Check sheet for the modelled part. Datum: model origin and axes. Units: mm. Give positions to 0.01 mm unless a question says otherwise; leave off trailing zeros. Order: outer loops, then holes, each group sorted by start corner. A loop starts at its lowest first (then second) coordinate and runs counter-clockwise, first axis right, second up. Notation, with made-up numbers: (28, -21) -> (55, -21) arc R27 ccw to (55, 6) -> close; hole circle Ø6 at (41, -30). An arc over 180 degrees is marked (long way). Answer in a Markdown table with one row per item. Add a question column.
(1) Cross-section at A-A (x = 10.5). Record the cut outline in (y, z).
(2) Cross-section at B-B (y = 21). Record the cut outline in (x, z), then the cut area to 3 significant figures.
(3) Cross-section at D-D (z = 0). Record the cut outline in (x, y).
(4) Release check for a two-part mould opening along Z. For faces 1 (the face through (22, 14, 0)), 2 (the face through (28.493, 14.297, 0.627)), 3 (the face through (0, 15, -25)) record: released by +Z, released by -Z, zero draft, split by the parting line, or undercut.
(5) Cross-section at C-C (x = 6.75). Record the cut outline in (y, z).
(6) Thickness scan on L1, parallel to Z at x = 7.75, y = 22.5; L2, parallel to Z at x = 17, y = 22.75; L3, parallel to X at y = 8.25, z = -17.5. Record the ranges inside material, lowest first. Write a range as [from, to].
(7) Go/stop test with flat-tipped pins: pin 1 (5 mm diameter, centred on y = 22, z = 3, fed in from +X); pin 2 (5 mm diameter, centred on x = 8, y = 9.5, fed in from +Z). Record where each tip stops, or that it passes through.
```python
from build123d import *

# Parameters (mm, degrees)
SKETCH1_R                = 28.5
SKETCH1_R_2              = 22
BOSS_EXTRUDE1_DEPTH      = 29
SPLIT1_SURFACE_1_BACK    = 86.668
SPLIT1_SURFACE_1_DEPTH   = 173.336
SPLIT1_SURFACE_2_BACK    = 86.668
SPLIT1_SURFACE_2_DEPTH   = 173.336
BODY_DELETE_KEEP_1_DEPTH = 29


# Read off the part's stored shape, not the designer's step: Body-Delete/Keep 1
with BuildPart() as part:
    # Sketch1 → Boss-Extrude1 (new body)
    with BuildSketch(Plane(origin=(0, 0, 0), x_dir=(1, 0, 0), z_dir=(0, 1, 0))):
        with Locations(Location((0, 0, 0), (0, 0, 270))):
            Circle(SKETCH1_R)
        with Locations(Location((0, 0, 0), (0, 0, 270))):
            Circle(SKETCH1_R_2, mode=Mode.SUBTRACT)
    extrude(amount=BOSS_EXTRUDE1_DEPTH)


with BuildPart() as body_2:
    # Split1: the piece behind the surface
    add(part.part)
    # Split1 surface: a surface, the sketch's curves swept straight by 173.336 mm
    with BuildLine(Plane.XY.offset(-SPLIT1_SURFACE_1_BACK), mode=Mode.PRIVATE) as split1_surface_1_path:
        Line((0, 33.955759062), (0, -6.102624859))
    split1_surface_1 = Shell.extrude(split1_surface_1_path.wire(), (0 * SPLIT1_SURFACE_1_DEPTH, 0 * SPLIT1_SURFACE_1_DEPTH, 1 * SPLIT1_SURFACE_1_DEPTH))
    split(bisect_by=split1_surface_1, keep=Keep.BOTTOM)

    # Body-Delete/Keep 1 outline → Body-Delete/Keep 1 (cut)
    with BuildSketch(Plane(origin=(0, 0, 0), x_dir=(1, 0, 0), z_dir=(0, 1, 0))):
        with BuildLine():
            Line((0, -28.5), (0, -22))
            ThreePointArc((0, -22), (-22, 0), (0, 22))
            Line((0, 22), (0, 28.5))
            ThreePointArc((0, 28.5), (-28.5, 0), (0, -28.5))
        make_face()
    extrude(amount=BODY_DELETE_KEEP_1_DEPTH, mode=Mode.SUBTRACT)


with BuildPart() as part_1:
    add(part.part)

    # Split1: split by a surface, the side it looks to stays
    # Split1 surface: a surface, the sketch's curves swept straight by 173.336 mm
    with BuildLine(Plane.XY.offset(-SPLIT1_SURFACE_2_BACK), mode=Mode.PRIVATE) as split1_surface_2_path:
        Line((0, 33.955759062), (0, -6.102624859))
    split1_surface_2 = Shell.extrude(split1_surface_2_path.wire(), (0 * SPLIT1_SURFACE_2_DEPTH, 0 * SPLIT1_SURFACE_2_DEPTH, 1 * SPLIT1_SURFACE_2_DEPTH))
    split(bisect_by=split1_surface_2, keep=Keep.TOP)


solid = part_1.part
```
Answer below:
| question | item | result |
|---|---|---|
| 1 | outline | (0, -26.5) -> (29, -26.5) -> (29, -19.33) -> (0, -19.33) -> close; (0, 19.33) -> (29, 19.33) -> (29, 26.5) -> (0, 26.5) -> close |
| 2 | outline | (0, -28.5) arc R28.5 ccw to (0, 28.5) -> (0, 22) arc R22 cw to (0, -22) -> close |
| 2 | area | 516 mm² |
| 3 | outline | (22, 0) -> (28.5, 0) -> (28.5, 29) -> (22, 29) -> close |
| 4 | face 1 | undercut |
| 4 | face 2 | split by the parting line |
| 4 | face 3 | zero draft |
| 5 | outline | (0, -27.69) -> (29, -27.69) -> (29, -20.94) -> (0, -20.94) -> close; (0, 20.94) -> (29, 20.94) -> (29, 27.69) -> (0, 27.69) -> close |
| 6 | L1 | z = [-27.43, -20.59], [20.59, 27.43] |
| 6 | L2 | z = [-22.87, -13.96], [13.96, 22.87] |
| 6 | L3 | x = [13.33, 22.49] |
| 7 | pin 1 | stops at x = 28.5 |
| 7 | pin 2 | stops at z = 27.96 |
